The listing builds one solid part. Answer for the finished solid, in the listing's coordinates (mm). Face numbers are marked on the shaded views. Coordinates: 2 decimals unless noted, no trailing zeros. Loops run counter-clockwise (first coordinate to the right, second up) from the corner with the lowest first, then second, coordinate; pieces in that order, holes last. Notation, with made-up numbers: M -19,36 L 30,36 A16 cw 30,54 Z; hole C 78.25,36.25 d4. An arc over 180 degrees is marked long. Answer in a Markdown table with one row per item. Add a question column.
from build123d import *

# Parameters (mm, degrees)
SKETCH1_W           = 76.2
SKETCH1_H           = 50.8
SKETCH1_R           = 3.175
SKETCH1_R_2         = 1.27
BOSS_EXTRUDE1_DEPTH = 3.175
FILLET1_R           = 10


with BuildPart() as part:
    # Sketch1 → Boss-Extrude1 (new body)
    with BuildSketch(Plane(origin=(0, 0, 0), x_dir=(1, 0, 0), z_dir=(0, 1, 0))):
        Rectangle(SKETCH1_W, SKETCH1_H)
        with Locations(Location((-25.4, 3.81, 0), (0, 0, 270))):
            Circle(SKETCH1_R, mode=Mode.SUBTRACT)
        with Locations(Location((25.4, 3.81, 0), (0, 0, 270))):
            Circle(SKETCH1_R, mode=Mode.SUBTRACT)
        with Locations(Location((0, 0, 0), (0, 0, 270))):
            Circle(SKETCH1_R_2, mode=Mode.SUBTRACT)
    extrude(amount=BOSS_EXTRUDE1_DEPTH)

    # Fillet1
    fillet1_edges = [part.edges().sort_by_distance(p)[0] for p in [
        (38.1, 1.5875, 25.4),
        (-38.1, 1.5875, 25.4),
        (-38.1, 1.5875, -25.4),
        (38.1, 1.5875, -25.4),
    ]]
    fillet(fillet1_edges, radius=FILLET1_R)


solid = part.part
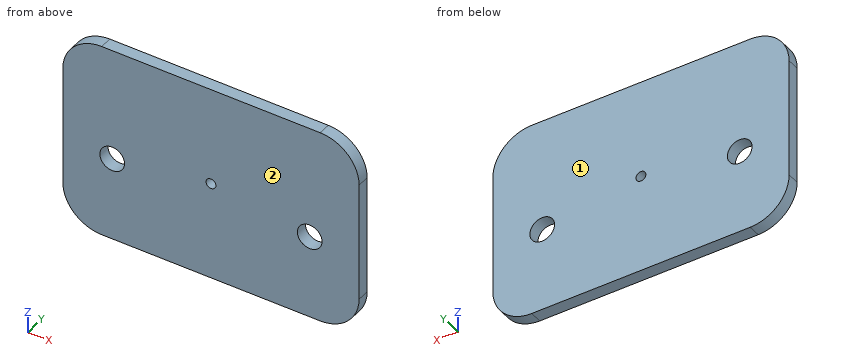
(1) A cutting plane is placed at D-D (x = 0). Give the vertices of the cut face in (y, z) (3 decimals).
(2) Straight lines are drawn through the part: line 1 (X direction, y = 1.75, z = -3.81) (3 decimals); line 2 (X direction, y = 2.35, z = 0); line 3 (Z direction, x = 23, y = 0.35). For each, find the intervals that lie inside material, in ascending order.
(3) The mould has two halves that part along Y. Classify the marked faces 1 and 2: released by +Y, released by -Y, zero draft, split by the parting line, or undercut.
(4) A cutting plane is placed at A-A (x = -25.4). Give the vertices of the cut face in (y, z) (3 decimals).
(5) A cutting plane is placed at C-C (y = 1.9). Give the vertices of the cut face in (x, z) (3 decimals).
(6) A cutting plane is placed at B-B (z = -3.81). Give the vertices of the cut face in (x, y) (3 decimals).
Solved:
| question | item | result |
|---|---|---|
| 1 | outline | M 0,-25.4 L 3.175,-25.4 L 3.175,-1.27 L 0,-1.27 Z; M 0,1.27 L 3.175,1.27 L 3.175,25.4 L 0,25.4 Z |
| 2 | line 1 | x = -38.1 to -28.575, -22.225 to 22.225, 28.575 to 38.1 |
| 2 | line 2 | x = -38.1 to -1.27, 1.27 to 38.1 |
| 2 | line 3 | z = -25.4 to -5.89, -1.73 to 25.4 |
| 3 | face 1 | released by +Y |
| 3 | face 2 | released by -Y |
| 4 | outline | M 0,-25.4 L 3.175,-25.4 L 3.175,-6.985 L 0,-6.985 Z; M 0,-0.635 L 3.175,-0.635 L 3.175,25.4 L 0,25.4 Z |
| 5 | outline | M -38.1,-15.4 A10 ccw -28.1,-25.4 L 28.1,-25.4 A10 ccw 38.1,-15.4 L 38.1,15.4 A10 ccw 28.1,25.4 L -28.1,25.4 A10 ccw -38.1,15.4 Z; hole C -25.4,-3.81 d6.35; hole C 0,0 d2.54; hole C 25.4,-3.81 d6.35 |
| 6 | outline | M -38.1,0 L -28.575,0 L -28.575,3.175 L -38.1,3.175 Z; M -22.225,0 L 22.225,0 L 22.225,3.175 L -22.225,3.175 Z; M 28.575,0 L 38.1,0 L 38.1,3.175 L 28.575,3.175 Z |
